from build123d import *

# Parameters (mm, degrees)
CYLINDER445_R               = 1.5
CYLINDER445_DEPTH           = 100
CYLINDER446_R               = 1.5
CYLINDER446_DEPTH           = 100
CYLINDER446_PLACEMENT_ANGLE = 135
CYLINDER447_R               = 1.5
CYLINDER447_DEPTH           = 100
CYLINDER448_R               = 1.5
CYLINDER448_DEPTH           = 100
CYLINDER448_PLACEMENT_ANGLE = 225
CYLINDER449_R               = 1.5
CYLINDER449_DEPTH           = 100
CYLINDER450_R               = 1.5
CYLINDER450_DEPTH           = 100
CYLINDER450_PLACEMENT_ANGLE = 45
CYLINDER451_R               = 1.5
CYLINDER451_DEPTH           = 100
CYLINDER444_R               = 1.5
CYLINDER444_DEPTH           = 100
CYLINDER444_PLACEMENT_ANGLE = 45
BOX154_W                    = 6
BOX154_H                    = 6
BOX154_DEPTH                = 10
BOX151_W                    = 6
BOX151_H                    = 6
BOX151_DEPTH                = 10
BOX155_W                    = 6
BOX155_H                    = 6
BOX155_DEPTH                = 10
BOX153_W                    = 6
BOX153_H                    = 6
BOX153_DEPTH                = 10
BOX156_W                    = 6
BOX156_H                    = 6
BOX156_DEPTH                = 10
BOX152_W                    = 6
BOX152_H                    = 6
BOX152_DEPTH                = 10
CYLINDER407_R               = 3
CYLINDER407_DEPTH           = 7
CYLINDER405_R               = 3
CYLINDER405_DEPTH           = 7
CYLINDER404_R               = 3
CYLINDER404_DEPTH           = 7
CYLINDER406_R               = 3
CYLINDER406_DEPTH           = 7
TUBE020_R                   = 58
TUBE020_R_2                 = 38
TUBE020_DEPTH               = 1


with BuildPart() as obj1:
    # Cylinder445 → Cylinder445 (new body)
    with BuildSketch(Plane(origin=(38.80294, -16.072704, 0), x_dir=(0, 1, 0), z_dir=(0, 0, 1))):
        Circle(CYLINDER445_R)
    extrude(amount=CYLINDER445_DEPTH)


with BuildPart() as obj2:
    # Cylinder446 → Cylinder446 (new body)
    with BuildSketch(Plane.XY):
        Circle(CYLINDER446_R)
    extrude(amount=CYLINDER446_DEPTH)


with BuildPart() as obj2_1:
    # Cylinder446 placement: moved
    add(obj2.part.moved(Location((38.80294, 16.072704, 0))).rotate(Axis((38.80294, 16.072704, 0), (0, 0, 1)), CYLINDER446_PLACEMENT_ANGLE))


with BuildPart() as obj3:
    # Cylinder447 → Cylinder447 (new body)
    with BuildSketch(Plane(origin=(16.072704, 38.80294, 0), x_dir=(-1, 0, 0), z_dir=(0, 0, 1))):
        Circle(CYLINDER447_R)
    extrude(amount=CYLINDER447_DEPTH)


with BuildPart() as obj4:
    # Cylinder448 → Cylinder448 (new body)
    with BuildSketch(Plane.XY):
        Circle(CYLINDER448_R)
    extrude(amount=CYLINDER448_DEPTH)


with BuildPart() as obj4_1:
    # Cylinder448 placement: moved
    add(obj4.part.moved(Location((-16.072704, 38.80294, 0))).rotate(Axis((-16.072704, 38.80294, 0), (0, 0, 1)), CYLINDER448_PLACEMENT_ANGLE))


with BuildPart() as obj5:
    # Cylinder449 → Cylinder449 (new body)
    with BuildSketch(Plane(origin=(-38.80294, 16.072704, 0), x_dir=(0, -1, 0), z_dir=(0, 0, 1))):
        Circle(CYLINDER449_R)
    extrude(amount=CYLINDER449_DEPTH)


with BuildPart() as obj6:
    # Cylinder450 → Cylinder450 (new body)
    with BuildSketch(Plane.XY):
        Circle(CYLINDER450_R)
    extrude(amount=CYLINDER450_DEPTH)


with BuildPart() as obj6_1:
    # Cylinder450 placement: moved
    add(obj6.part.moved(Location((-38.80294, -16.072704, 0))).rotate(Axis((-38.80294, -16.072704, 0), (0, 0, -1)), CYLINDER450_PLACEMENT_ANGLE))


with BuildPart() as obj7:
    # Cylinder451 → Cylinder451 (new body)
    with BuildSketch(Plane(origin=(-16.072704, -38.80294, 0), x_dir=(1, 0, 0), z_dir=(0, 0, 1))):
        Circle(CYLINDER451_R)
    extrude(amount=CYLINDER451_DEPTH)


with BuildPart() as compound325:
    # Cylinder444 → Cylinder444 (new body)
    with BuildSketch(Plane.XY):
        Circle(CYLINDER444_R)
    extrude(amount=CYLINDER444_DEPTH)


with BuildPart() as compound325_1:
    # Cylinder444 placement: moved
    add(compound325.part.moved(Location((16.072704, -38.80294, 0))).rotate(Axis((16.072704, -38.80294, 0), (0, 0, 1)), CYLINDER444_PLACEMENT_ANGLE))

    # Compound325: union obj1, obj2, obj3, obj4, obj5, obj6, obj7
    add(obj1.part)
    add(obj2_1.part)
    add(obj3.part)
    add(obj4_1.part)
    add(obj5.part)
    add(obj6_1.part)
    add(obj7.part)


with BuildPart() as krychle154:
    # Box154 → Box154 (new body)
    with BuildSketch(Plane(origin=(-37, -39, 40), x_dir=(1, 0, 0), z_dir=(0, 0, 1))):
        with Locations((3, 3)):
            Rectangle(BOX154_W, BOX154_H)
    extrude(amount=BOX154_DEPTH)


with BuildPart() as krychle151:
    # Box151 → Box151 (new body)
    with BuildSketch(Plane(origin=(-3, -53, 40), x_dir=(1, 0, 0), z_dir=(0, 0, 1))):
        with Locations((3, 3)):
            Rectangle(BOX151_W, BOX151_H)
    extrude(amount=BOX151_DEPTH)


with BuildPart() as krychle155:
    # Box155 → Box155 (new body)
    with BuildSketch(Plane(origin=(31, 33, 40), x_dir=(1, 0, 0), z_dir=(0, 0, 1))):
        with Locations((3, 3)):
            Rectangle(BOX155_W, BOX155_H)
    extrude(amount=BOX155_DEPTH)


with BuildPart() as krychle153:
    # Box153 → Box153 (new body)
    with BuildSketch(Plane(origin=(-37, 33, 40), x_dir=(1, 0, 0), z_dir=(0, 0, 1))):
        with Locations((3, 3)):
            Rectangle(BOX153_W, BOX153_H)
    extrude(amount=BOX153_DEPTH)


with BuildPart() as krychle156:
    # Box156 → Box156 (new body)
    with BuildSketch(Plane(origin=(31, -39, 40), x_dir=(1, 0, 0), z_dir=(0, 0, 1))):
        with Locations((3, 3)):
            Rectangle(BOX156_W, BOX156_H)
    extrude(amount=BOX156_DEPTH)


with BuildPart() as compound316:
    # Box152 → Box152 (new body)
    with BuildSketch(Plane(origin=(-3, 47, 40), x_dir=(1, 0, 0), z_dir=(0, 0, 1))):
        with Locations((3, 3)):
            Rectangle(BOX152_W, BOX152_H)
    extrude(amount=BOX152_DEPTH)

    # Compound316: union Krychle154, Krychle151, Krychle155, Krychle153, Krychle156
    add(krychle154.part)
    add(krychle151.part)
    add(krychle155.part)
    add(krychle153.part)
    add(krychle156.part)


with BuildPart() as compound316_1:
    # Compound316 placement: moved
    add(compound316.part.moved(Location((0, 0, -18))))


with BuildPart() as obj8:
    # Cylinder407 → Cylinder407 (new body)
    with BuildSketch(Plane(origin=(51, -16, 50), x_dir=(1, 0, 0), z_dir=(0, 0, 1))):
        Circle(CYLINDER407_R)
    extrude(amount=CYLINDER407_DEPTH)


with BuildPart() as obj9:
    # Cylinder405 → Cylinder405 (new body)
    with BuildSketch(Plane(origin=(51, 7, 50), x_dir=(1, 0, 0), z_dir=(0, 0, 1))):
        Circle(CYLINDER405_R)
    extrude(amount=CYLINDER405_DEPTH)


with BuildPart() as obj10:
    # Cylinder404 → Cylinder404 (new body)
    with BuildSketch(Plane(origin=(-51, 7, 50), x_dir=(1, 0, 0), z_dir=(0, 0, 1))):
        Circle(CYLINDER404_R)
    extrude(amount=CYLINDER404_DEPTH)


with BuildPart() as compound312:
    # Cylinder406 → Cylinder406 (new body)
    with BuildSketch(Plane(origin=(-51, -16, 50), x_dir=(1, 0, 0), z_dir=(0, 0, 1))):
        Circle(CYLINDER406_R)
    extrude(amount=CYLINDER406_DEPTH)

    # Compound312: union obj8, obj9, obj10
    add(obj8.part)
    add(obj9.part)
    add(obj10.part)


with BuildPart() as compound312_1:
    # Compound312 placement: moved
    add(compound312.part.moved(Location((0, 0, -25))))


with BuildPart() as cut173:
    # Tube020 → Tube020 (new body)
    with BuildSketch(Plane.XY.offset(31)):
        Circle(TUBE020_R)
        Circle(TUBE020_R_2, mode=Mode.SUBTRACT)
    extrude(amount=TUBE020_DEPTH)

    # Cut161: cut Compound312
    add(compound312_1.part, mode=Mode.SUBTRACT)

    # Cut163: cut Compound316
    add(compound316_1.part, mode=Mode.SUBTRACT)

    # Cut173: cut Compound325
    add(compound325_1.part, mode=Mode.SUBTRACT)


solid = cut173.part
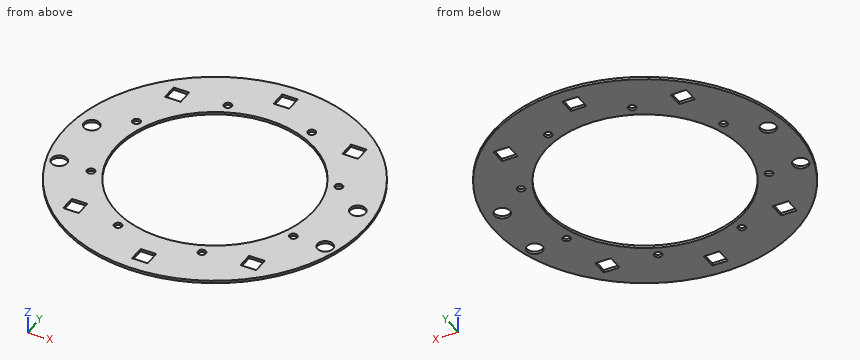
For this review, take the finished solid that the model builds, in its own axes (mm). Round coordinates to 2 decimals unless told otherwise and drop trailing zeros. Loops run counter-clockwise (first coordinate to the right, second up) from the corner with the lowest first, then second, coordinate; pieces in that order, holes last. Notation, with made-up numbers: (22.25, 86) - (78.25, 86) arc R13 cw to (78.25, 92) - close; hole circle Ø8 at (-7, 83.25). An arc over 180 degrees is marked (long way). Use one line per item in the form item = value.
1) Clearance check with flat-ended pins moving along their axes: P1, Ø3.5, axis at x = 51, y = -16, coming from the -Z side; P2, Ø0.5, axis at x = -33, z = 31.5, coming from the +Y side; P3, Ø0.5, axis at y = -36, z = 31.5, coming from the +X side. State where each tip first meets the part, or that it passes through.
Solutions:
P1 = through
P2 = 47.87
P3 = 45.67
2) We need section D-D on y = 7. Write out the cut boundary in (x, z).
Solutions:
outline = (-57.58, 31) - (-54, 31) - (-54, 32) - (-57.58, 32) - close; (-48, 31) - (-37.35, 31) - (-37.35, 32) - (-48, 32) - close; (37.35, 31) - (48, 31) - (48, 32) - (37.35, 32) - close; (54, 31) - (57.58, 31) - (57.58, 32) - (54, 32) - close
3) We need section A-A on x = 0. Write out the cut boundary in (y, z).
Solutions:
outline = (-58, 31) - (-53, 31) - (-53, 32) - (-58, 32) - close; (-47, 31) - (-38, 31) - (-38, 32) - (-47, 32) - close; (38, 31) - (47, 31) - (47, 32) - (38, 32) - close; (53, 31) - (58, 31) - (58, 32) - (53, 32) - close
4) We need section C-C on x = 51. Write out the cut boundary in (y, z), then the cut area to 3 significant figures.
Solutions:
outline = (-27.62, 31) - (-19, 31) - (-19, 32) - (-27.62, 32) - close; (-13, 31) - (4, 31) - (4, 32) - (-13, 32) - close; (10, 31) - (27.62, 31) - (27.62, 32) - (10, 32) - close
area = 43.2 mm2
5) Wall thickness on probe 1 along X at (y, z) = (-16, 31.4); probe 2 along Y at (x, z) = (17, 31.7); probe 3 along X at (y, z) = (-1.5, 31.9): over which ranges is each line inside the solid? List them lowest first.
Solutions:
probe_1 = -55.75 to -54, -48 to -40.3, -37.3 to -34.47, 34.47 to 37.3, 40.3 to 48, 54 to 55.75
probe_2 = -55.45 to -39.98, -37.62 to -33.99, 33.99 to 37.62, 39.98 to 55.45
probe_3 = -57.98 to -37.97, 37.97 to 57.98
6) We need section B-B on y = -31. Write out the cut boundary in (x, z).
Solutions:
outline = (-49.02, 31) - (-21.98, 31) - (-21.98, 32) - (-49.02, 32) - close; (21.98, 31) - (49.02, 31) - (49.02, 32) - (21.98, 32) - close
